```python
from build123d import *

# Parameters (mm, degrees)
F0_W      = 457.2
F0_H      = 67.7333333333
F1_DEPTH  = 44.45
F10_DEPTH = 33.782


with BuildPart() as f1:
    # F0 (on Top) → F1 (new body)
    with BuildSketch(Plane.XY):
        Polygon((-228.6, 203.2), (-330.2, 203.2), (-330.2, -203.2), (-228.6, -203.2), (-228.6, -135.4666666667), (-228.6, -67.7333333333), (-228.6, 0), (-228.6, 67.7333333333), (-228.6, 135.4666666667), align=None)
        with Locations((0, -169.3333333333)):
            Rectangle(F0_W, F0_H)
        with Locations((0, -101.6)):
            Rectangle(F0_W, F0_H)
        with Locations((0, -33.8666666667)):
            Rectangle(F0_W, F0_H)
        with Locations((0, 33.8666666667)):
            Rectangle(F0_W, F0_H)
        with Locations((0, 101.6)):
            Rectangle(F0_W, F0_H)
        with Locations((0, 169.3333333333)):
            Rectangle(F0_W, F0_H)
        Polygon((330.2, 203.2), (228.6, 203.2), (228.6, 135.4666666667), (228.6, 67.7333333333), (228.6, 0), (228.6, -67.7333333333), (228.6, -135.4666666667), (228.6, -203.2), (330.2, -203.2), align=None)
    extrude(amount=F1_DEPTH)

    # F4: sweep along a path in F2
    with BuildLine(Plane.XY.offset(44.45)) as f4_path:
        Line((-228.6, 203.2), (-228.6, -203.2))
    # F3 (on face) → F4 (sweep, cut)
    with BuildSketch(Plane.XZ.offset(203.2)):
        Polygon((-226.06, 44.45), (-228.6, 44.45), (-231.14, 44.45), (-228.6, 41.91), align=None)
        Polygon((228.6, 44.45), (226.06, 44.45), (228.6, 41.91), (231.14, 44.45), align=None)
    sweep(path=f4_path.line, mode=Mode.SUBTRACT)

    # F8: sweep along a path in F6
    with BuildLine(Plane.XY.offset(44.45)) as f8_path:
        Line((-226.06, -67.7333333333), (226.06, -67.7333333333))
    # F7 (on offset) → F8 (sweep, cut)
    with BuildSketch(Plane.YZ.offset(228.6)):
        Polygon((-132.9266666667, 44.45), (-135.4666666667, 44.45), (-138.0066666667, 44.45), (-135.4666666667, 41.91), align=None)
        Polygon((-67.7333333333, 44.45), (-70.2733333333, 44.45), (-67.7333333333, 41.91), (-65.1933333333, 44.45), align=None)
        Polygon((0, 44.45), (-2.54, 44.45), (0, 41.91), (2.54, 44.45), align=None)
        Polygon((67.7333333333, 44.45), (65.1933333333, 44.45), (67.7333333333, 41.91), (70.2733333333, 44.45), align=None)
        Polygon((135.4666666667, 44.45), (132.9266666667, 44.45), (135.4666666667, 41.91), (138.0066666667, 44.45), align=None)
    sweep(path=f8_path.line, mode=Mode.SUBTRACT)

    # F9 (on face) → F10 (cut)
    with BuildSketch(Plane.XZ.offset(203.2)):
        Polygon((-173.269695488, 0), (-151.3092788213, 44.45), (-203.2, 44.45), (-199.7604166667, 0), align=None)
        Polygon((203.2, 44.45), (151.3092788213, 44.45), (173.269695488, 0), (199.7604166667, 0), align=None)
    extrude(amount=-F10_DEPTH, mode=Mode.SUBTRACT)


solid = f1.part
```
Verification items for the finished model (mm, model axes). A direction names the side the tool comes from. Give positions to 0.01 mm unless a question says otherwise; leave off trailing zeros.
1. Mould release check, pull along X, two halves, no side actions. Record for faces 1 (the flat face through (-330.2, 3, 22)), 2 (the flat face through (-162.443, -186.545, 21.914)), 3 (the flat face through (-5, 3, 0)): released by +X, released by -X, zero draft, split by the parting line, or undercut.
2. Set-up check for faces 4 (the flat face through (264, -203.2, 22)), 5 (the flat face through (201.456, -186.545, 21.914)): record each of +Z, -Z, +X, -X, +Y, -Y from which the full face is reachable in a straight line by a thin tool's end or side.
3. Thickness scan on line 1 (X direction, y = -173.5, z = 16.5); line 2 (Y direction, x = -216, z = 42); line 3 (X direction, y = -176.5, z = 31). Record the ranges inside material, lowest first.
Geometry says:
1. face 1: released by -X
1. face 2: undercut
1. face 3: zero draft
2. face 4: +Z, -Z, +X, -X, -Y
2. face 5: +Z, -Y
3. line 1: x = -330.2 to -201.04, -165.12 to 165.12, 201.04 to 330.2
3. line 2: y = -203.2 to -135.56, -135.38 to -67.82, -67.64 to -0.09, 0.09 to 67.64, 67.82 to 135.38, 135.56 to 203.2
3. line 3: x = -330.2 to -202.16, -157.95 to 157.95, 202.16 to 330.2
